from build123d import *

# Parameters (mm, degrees)
EXTRUSION1_DEPTH = 30
ESQUISSE2_R      = 1.5
ESQUISSE2_W      = 11.5
ESQUISSE2_H      = 7
EXTRUSION2_DEPTH = 30


with BuildPart() as part:
    # Esquisse1 → Extrusion1 (new body)
    with BuildSketch(Plane.XY):
        Polygon((-276.465646311, 896.941960338), (-276.465646311, 911.941960338), (-289.465646311, 911.941960338), (-289.465646311, 910.441960338), (-277.965646311, 910.441960338), (-277.965646311, 896.941960338), align=None)
    extrude(amount=EXTRUSION1_DEPTH)

    # Esquisse2 → Extrusion2 (cut)
    with BuildSketch(Plane(origin=(0, 911.941960338, 0), x_dir=(-1, 0, 0), z_dir=(0, 1, 0))):
        with Locations(Location((285.465646311, 16, 0), (0, 0, 90))):
            Circle(ESQUISSE2_R)
        with Locations(Location((285.465646311, 26, 0), (0, 0, 90))):
            Circle(ESQUISSE2_R)
        with Locations((283.715646311, 3.5)):
            Rectangle(ESQUISSE2_W, ESQUISSE2_H)
    extrude(amount=-EXTRUSION2_DEPTH, mode=Mode.SUBTRACT)


solid = part.part
Work out the finished part from the listing and answer in its coordinate system (mm). A direction names the side the tool comes from. Coordinates: 2 decimals unless noted, no trailing zeros. Loops run counter-clockwise (first coordinate to the right, second up) from the corner with the lowest first, then second, coordinate; pieces in that order, holes last. Notation, with made-up numbers: M -29.5,-14.75 L -10.5,-14.75 A6 ccw -10.5,-6.75 Z; hole C -25,19 d1. An arc over 180 degrees is marked long. Answer in a Markdown table with one row per item. Add a question column.
1. Flat-ended cylindrical pins translate along their axes: P1, Ø2.5, axis at x = -285.47, z = 16, coming from the +Y side; P2, Ø4, axis at y = 905.5, z = 13.5, coming from the -X side; P3, Ø4, axis at x = -282, y = 909, coming from the -Z side. Find the tip coordinate at first contact, or state that the pin passes through.
2. Find section D-D, the plane y = 907. Write down the section's boundary in (x, z).
3. Consider L1, parallel to X at y = 911.2, z = 26; L2, parallel to X at y = 907.25, z = 4.25; L3, parallel to Y at x = -284.25, z = 13.5. Determine where each line is inside the solid, lowest interval first.
4. The mould has two halves that part along Z. Classify faces 4 (the flat face through (-277, 905, 0)), 5 (the flat face through (-289.466, 911, 18)), 6 (the cylindrical face through (-283.98, 911.2, 25.8)): pulls with the +Z half, pulls with the -Z half, needs draft (parallel to the pull), parting line crosses it, or undercut.
5. A tool of negligible diameter and unlimited length cuts with its end or side. For faces 1 (the flat face through (-284, 911, 7)), 2 (the flat face through (-283, 911.942, 18)), 3 (the flat face through (-284, 910.442, 18)), from which of +Z, -Z, +X, -X, +Y, -Y can it reach the whole face along a straight path? Write none if from no direction.
6. Find section C-C, the plane z = 22.5. Write down the section's boundary in (x, y).
7. Find section A-A, the plane z = 26. Write down the section's boundary in (x, y), then the cut area to 4 significant figures.
8. Find section B-B, the plane x = -285. Write down the section's boundary in (y, z).
Reported:
| question | item | result |
|---|---|---|
| 1 | P1 | passes through |
| 1 | P2 | stops at x = -277.97 |
| 1 | P3 | stops at z = 7 |
| 2 | outline | M -277.97,0 L -276.47,0 L -276.47,30 L -277.97,30 Z |
| 3 | L1 | x = -289.47 to -286.97, -283.97 to -276.47 |
| 3 | L2 | x = -277.97 to -276.47 |
| 3 | L3 | y = 910.44 to 911.94 |
| 4 | face 4 | pulls with the -Z half |
| 4 | face 5 | needs draft |
| 4 | face 6 | undercut |
| 5 | face 1 | -Z, -X, +Y, -Y |
| 5 | face 2 | +Z, -Z, +X, -X, +Y |
| 5 | face 3 | +Z, -Z, -X, -Y |
| 6 | outline | M -289.47,910.44 L -277.97,910.44 L -277.97,896.94 L -276.47,896.94 L -276.47,911.94 L -289.47,911.94 Z |
| 7 | outline | M -289.47,910.44 L -286.97,910.44 L -286.97,911.94 L -289.47,911.94 Z; M -283.97,910.44 L -277.97,910.44 L -277.97,896.94 L -276.47,896.94 L -276.47,911.94 L -283.97,911.94 Z |
| 7 | area | 35.25 mm^2 |
| 8 | outline | M 910.44,7 L 911.94,7 L 911.94,14.57 L 910.44,14.57 Z; M 910.44,17.43 L 911.94,17.43 L 911.94,24.57 L 910.44,24.57 Z; M 910.44,27.43 L 911.94,27.43 L 911.94,30 L 910.44,30 Z |
